```python
from build123d import *

# Parameters (mm, degrees)
SKETCH2_W           = 3.25
SKETCH2_H           = 3.25
CUT_EXTRUDE1_DEPTH  = 7
CUT_EXTRUDE2_START  = -20
SKETCH3_R           = 5
CUT_EXTRUDE2_DEPTH  = 20
CHAMFER1_SIZE       = 0.3
BOSS_EXTRUDE1_START = -3
SKETCH5_R           = 7
BOSS_EXTRUDE1_DEPTH = 3
CHAMFER2_SIZE       = 0.3


with BuildPart() as part:
    # Sketch1 → Revolve1 (revolve)
    with BuildSketch(Plane.XY, mode=Mode.PRIVATE) as revolve1_sk:
        Polygon((0, 0), (5, 0), (5, 70), (7, 70), (7, 73), (5, 73), (5, 81), (0, 81), align=None)
    revolve(revolve1_sk.sketch.rotate(Axis((0, 81, 0), (0, -1, 0)), 180), axis=Axis((0, 81, 0), (0, -1, 0)))

    # Sketch2 → Cut-Extrude1 (cut)
    with BuildSketch(Plane.XZ.offset(-70)):
        with Locations((0, 5)):
            Rectangle(SKETCH2_W, SKETCH2_H)
    extrude(amount=CUT_EXTRUDE1_DEPTH, mode=Mode.SUBTRACT)

    # Sketch3 → Cut-Extrude2 (cut)
    with BuildSketch(Plane.XZ.offset(CUT_EXTRUDE2_START)):
        with Locations(Location((0, 0, 0), (0, 0, 108.965574989))):
            Circle(SKETCH3_R)
        with BuildLine():
            ThreePointArc((1.125, 3.838538133), (0, -4), (-1.125, 3.838538133))
            Line((-1.125, 3.838538133), (-1.125, 2.875))
            Line((-1.125, 2.875), (1.125, 2.875))
            Line((1.125, 2.875), (1.125, 3.838538133))
        make_face(mode=Mode.SUBTRACT)
    extrude(amount=CUT_EXTRUDE2_DEPTH, mode=Mode.SUBTRACT)

    # Chamfer1
    chamfer1_edges = [part.edges().sort_by_distance(p)[0] for p in [
        (-1.125, 0, 3.356769067),
        (0, 0, 2.875),
        (0, 0, -4),
        (1.125, 0, 3.356769067),
        (5, 81, 0),
        (7, 73, 0),
        (7, 70, 0),
    ]]
    chamfer(chamfer1_edges, length=CHAMFER1_SIZE)

    # Sketch5 → Boss-Extrude1 (add)
    with BuildSketch(Plane(origin=(0, 26, 0), x_dir=(-1, 0, 0), z_dir=(0, -1, 0)).offset(BOSS_EXTRUDE1_START)):
        Circle(SKETCH5_R)
    extrude(amount=BOSS_EXTRUDE1_DEPTH)

    # Chamfer2
    chamfer2_edges = [part.edges().sort_by_distance(p)[0] for p in [
        (7, 29, 0),
        (7, 26, 0),
    ]]
    chamfer(chamfer2_edges, length=CHAMFER2_SIZE)


solid = part.part
```
Read the model definition and answer for the solid it produces. Units are mm, in the model's axes. A direction names the side the tool comes from. Give positions to 0.01 mm unless a question says otherwise; leave off trailing zeros. Write each loop counter-clockwise with the first axis right and the second up, starting at its lowest first coordinate (ties: lowest second). Pieces come first, ordered by that corner, then holes. Notation, with made-up numbers: (55, -25.75) - (73, -25.75) arc R21 ccw to (73, -17.75) - close; hole circle Ø4 at (4, -30.75). An arc over 180 degrees is marked (long way). Write item = value, one per line. Start each with the question number.
Item 1: The mould has two halves that part along X. Classify faces 5 (the flat face through (1.625, 67, 4)), 6 (the cylindrical face through (-3, 50, -4)), 7 (the flat face through (0, 81, 0)), 8 (the flat face through (-1.625, 67, 4)): +X half, -X half, draft (parallel to the pull), parting line (faces both ways), or undercut.
Item 2: Find section A-A (y = 72). Give the vertices of the cut face in (x, z), then the cut area to 3 significant figures.
Item 3: A tool of negligible diameter and unlimited length cuts with its end or side. For faces 1 (the flat face through (0, 67, 3.375)), 2 (the cylindrical face through (0, 10, -4)), 3 (the cylindrical face through (5, 77, 0)), 4 (the flat face through (0, 70, 4)), from which of +Z, -Z, +X, -X, +Y, -Y can it reach the whole face along a straight path? Write none if from no direction.
Item 4: Each of these flat-tipped pins is pushed along its axis until it touches: P1, Ø3, axis at y = 21, z = -5.5, coming from the -X side; P2, Ø3, axis at x = 3.5, y = 43, coming from the +Z side; P3, Ø1.1, axis at x = 0.5, y = 13.5, coming from the +Z side (3 decimals); P4, Ø5, axis at y = 73, z = -2, coming from the +X side. Where does it stop, or does it pass through?
Item 5: Find the intervals of material crossed by probe 1 along Y at (x, z) = (-4, 4.5); probe 2 along X at (y, z) = (18, 1.5); probe 3 along Z at (x, y) = (3, 54), in increasing order. Write a range as [from, to].
Item 6: Find section B-B (y = 24.5). Give the vertices of the cut face in (x, z).
Response:
q1.face_5 = undercut
q1.face_6 = parting line
q1.face_7 = draft
q1.face_8 = undercut
q2.outline = circle Ø14 at (0, 0)
q2.area = 154 mm²
q3.face_1 = +Z
q3.face_2 = -Y
q3.face_3 = +Y
q3.face_4 = none
q4.P1 = -3
q4.P2 = 4.58
q4.P3 = 2.875
q4.P4 = 7
q5.probe_1 = [26, 29], [70, 73]
q5.probe_2 = [-3.71, 3.71]
q5.probe_3 = [-4, 4]
q6.outline = circle Ø10 at (0, 0)
